Input: part model. Units: mm. Frame: model coordinates. Give positions to 0.01 mm unless a question says otherwise; leave off trailing zeros. Loops run counter-clockwise (first coordinate to the right, second up) from the corner with the lowest first, then second, coordinate; pieces in that order, holes last. Notation, with made-up numbers: M 23,48.25 L 77,48.25 A26 ccw 77,73.25 Z; hole C -3.75,-25.5 d5. An arc over 180 degrees is marked long. Answer as a JSON object with one key per item and string values. Group by question number.
1) Ray query, L1, parallel to X at y = 6, z = -15; L2, parallel to Y at x = 90, z = 11; L3, parallel to Y at x = 136, z = -1.5. Return the intervals inside material, ascending.
2) First-contact query: P1, Ø1, axis at x = 128.5, z = 7.5, coming from the -Y side; P2, Ø12, axis at x = 27, y = -9, coming from the +Z side; P3, Ø3, axis at x = 26.5, z = 8, coming from the +Y side; P4, Ø1.5, axis at y = -9.5, z = -13.5, coming from the +X side. Flat tips, straight axial feed; report the tip coordinate or a pass-through.
3) Section query A-A on x = 53.5. Return loops of the section in (y, z), plus the area to 3 significant figures.
from build123d import *

# Parameters (mm, degrees)
HEADCHAMFER_SIZE = 2.165


with BuildPart() as part:
    # Sketch1 → Base (revolve)
    with BuildSketch(Plane.XY, mode=Mode.PRIVATE) as base_sk:
        Polygon((0, 0), (0, 18), (78, 18), (84, 16.701), (116, 16.701), (122, 18), (200, 18), (200, 0), align=None)
    revolve(base_sk.sketch.rotate(Axis((-1.310841664, 0, 0), (1, 0, 0)), 90), axis=Axis((-1.310841664, 0, 0), (1, 0, 0)))

    # HeadChamfer
    headchamfer_edges = [part.edges().sort_by_distance(p)[0] for p in [
        (200, 0, -18),
        (0, 0, -18),
    ]]
    chamfer(headchamfer_edges, length=HEADCHAMFER_SIZE)

    # Sketch4 → BaseBody (revolve)
    with BuildSketch(Plane.XY, mode=Mode.PRIVATE) as basebody_sk:
        Polygon((78, 16.701), (84, 18), (116, 18), (122, 16.701), align=None)
    revolve(basebody_sk.sketch.rotate(Axis((-7.809086942, 0, 0), (1, 0, 0)), 90), axis=Axis((-7.809086942, 0, 0), (1, 0, 0)))


solid = part.part
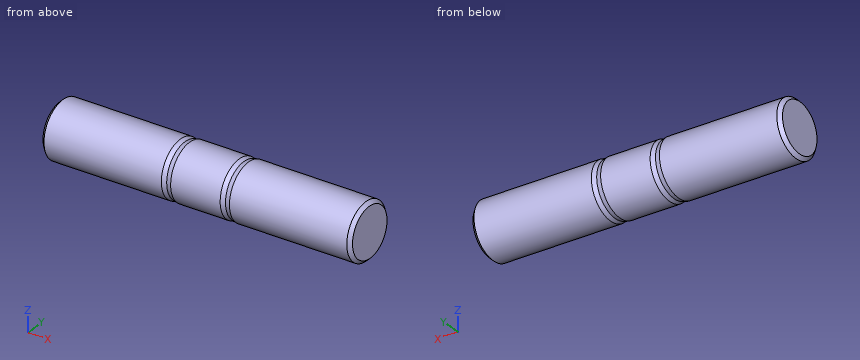
Output:
{
 "1": {"L1": "x = 0.32 to 199.68", "L2": "y = -14.25 to 14.25", "L3": "y = -17.94 to 17.94"},
 "2": {"P1": "stops at y = -16.58", "P2": "stops at z = 17.75", "P3": "stops at y = 16.79", "P4": "stops at x = 200"},
 "3": {"outline": "C 0,0 d36", "area": "1,020 mm^2"}
}
